For this review, take the finished solid that the model builds, in its own axes (mm). Face numbers are marked on the shaded views. A direction names the side the tool comes from. Round coordinates to 2 decimals unless told otherwise and drop trailing zeros. Order: outer loops, then holes, each group sorted by start corner. A loop starts at its lowest first (then second) coordinate and runs counter-clockwise, first axis right, second up. Notation, with made-up numbers: (2.5, 86) -> (17.5, 86) arc R14 cw to (17.5, 113) -> close; hole circle Ø4 at (-32, 38.5). An arc over 180 degrees is marked (long way). Put each result on its own line as item: value. Start each with the question number.
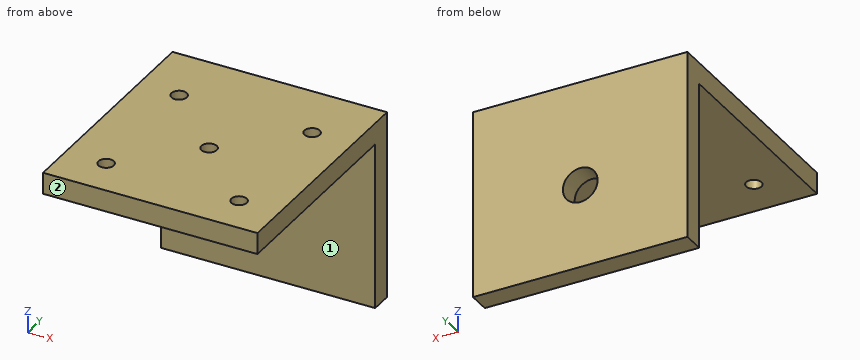
Autodesk Inventor part; units mm, degrees
ref_plane "YZ Plane" through (0, 0, 0) normal (1, 0, 0) x (0, 1, 0)
ref_plane "XZ Plane" through (0, 0, 0) normal (0, 1, 0) x (-1, 0, 0)
ref_plane "XY Plane" through (0, 0, 0) normal (0, 0, 1) x (1, 0, 0)
sketch "Эскиз1" plane through (0, 0, 0) normal (0, 0, 1) x (1, 0, 0)
  line L0 (-25, -25) -> (25, -25)
  line L1 (25, -25) -> (25, 25)
  line L2 (25, 25) -> (-25, 25)
  line L3 (-25, 25) -> (-25, -25)
  circle A0 centre (0, 0) radius 1.8
  circle A1 centre (15.5, 15.5) radius 1.8
  circle A2 centre (-15.5, 15.5) radius 1.8
  circle A3 centre (-15.5, -15.5) radius 1.8
  circle A4 centre (15.5, -15.5) radius 1.8
  dimension "d0" = 50
  dimension "d1" = 50
  dimension "d2" = 3.6
  dimension "d3" = 3.6
  dimension "d6" = 360
  dimension "d14" = 25
  dimension "d15" = 25
  dimension "d16" = 9.5
  dimension "d17" = 9.5
extrude "Выдавливание1" add sketch "Эскиз1" along normal blind 5
sketch "Эскиз2" plane through (-25, 25, 0) normal (0, 1, 0) x (1, 0, 0)
  line L0 (0, 0) -> (50, 0)
  line L1 (50, 0) -> (50, 39)
  line L2 (50, 39) -> (0, 39)
  line L3 (0, 39) -> (0, 0)
  line L4 (0, -5) -> (50, -5)
  line L5 (50, 0) -> (50, -5)
  line L6 (0, -5) -> (50, -5)
  line L7 (50, -5) -> (50, 0)
  line L8 (50, 0) -> (0, 0)
  line L9 (0, 0) -> (0, -5)
  circle A0 centre (25, 19.5) radius 4.05
  point P0 (25, 0)
  dimension "d10" = 50
  dimension "d11" = 39
  dimension "d19" = 8.1
extrude "Выдавливание3" add sketch "Эскиз2" along normal blind 5
properties part number "non_motor_holder"
Item 1: Consider section C-C, the plane y = 15.5. Write out the cut boundary in (x, z).
Item 2: Tool access review of the marked faces 1 and 2: name each direction out of +Z, -Z, +X, -X, +Y, -Y from which nothing blocks a thin tool from reaching the whole face with its end or side.
Item 3: Consider section A-A, the plane z = -19.5. Write out the cut boundary in (x, y), plus the area to 4 significant figures.
Item 4: Consider section D-D, the plane y = 0. Write out the cut boundary in (x, z).
Item 5: For L1, parallel to Y at x = -15.5, z = 2.2; L2, parallel to Y at x = -15, z = 1; L3, parallel to Y at x = -1, z = -28, list the stretches that pass through material, from the lowest coordinate up.
Item 6: Insertion check: pin 1 Ø4 at (x, z) = (-16.5, -5) entering from -Y; pin 2 Ø2 at (x, y) = (15.5, -15.5) entering from +Z; pin 3 Ø6 at (x, y) = (15.5, 15.5) entering from +Z; pin 4 Ø5 at (x, y) = (5.5, 15.5) entering from -Z. Each pin has a flat end and moves straight along its axis. Give the tip position at first contact, or say it passes through.
Item 7: Consider section B-B, the plane x = 15.5. Write out the cut boundary in (y, z).
Evaluation:
1. outline: (-25, 0) -> (-17.3, 0) -> (-17.3, 5) -> (-25, 5) -> close; (-13.7, 0) -> (13.7, 0) -> (13.7, 5) -> (-13.7, 5) -> close; (17.3, 0) -> (25, 0) -> (25, 5) -> (17.3, 5) -> close
2. face 1: -Z, +X, -X, -Y
2. face 2: +Z, -Z, +X, -X, -Y
3. outline: (-25, 25) -> (-4.05, 25) -> (-4.05, 30) -> (-25, 30) -> close; (4.05, 25) -> (25, 25) -> (25, 30) -> (4.05, 30) -> close
3. area: 209.5 mm^2
4. outline: (-25, 0) -> (-1.8, 0) -> (-1.8, 5) -> (-25, 5) -> close; (1.8, 0) -> (25, 0) -> (25, 5) -> (1.8, 5) -> close
5. L1: y = -25 to -17.3, -13.7 to 13.7, 17.3 to 30
5. L2: y = -25 to -17.23, -13.77 to 13.77, 17.23 to 30
5. L3: y = 25 to 30
6. pin 1: stops at y = 25
6. pin 2: passes through
6. pin 3: stops at z = 5
6. pin 4: stops at z = 0
7. outline: (-25, 0) -> (-17.3, 0) -> (-17.3, 5) -> (-25, 5) -> close; (-13.7, 0) -> (13.7, 0) -> (13.7, 5) -> (-13.7, 5) -> close; (17.3, 0) -> (25, 0) -> (25, -39) -> (30, -39) -> (30, 5) -> (17.3, 5) -> close
